from build123d import *

# Parameters (mm, degrees)
EXTRUDE_THIN1_DEPTH      = 5
EXTRUDE_THIN1_DEPTH_BACK = 1


with BuildPart() as part:
    # Sketch1 → Extrude-Thin1 (new, two sides: drawn at the far end of the back side and taken through both)
    with BuildSketch(Plane(origin=(0, 494, 0), x_dir=(1, 0, 0), z_dir=(0, 1, 0)).offset(-EXTRUDE_THIN1_DEPTH_BACK)):
        with BuildLine():
            Line((-21.192485275, 22.077376905), (159.5, 22.077376905))
            ThreePointArc((159.5, 22.077376905), (164.149331935, 20.119811555), (165.998241995, 15.426211538))
            Line((165.998241995, 15.426211538), (160.501622773, -220.860462738))
            ThreePointArc((160.501622773, -220.860462738), (166.44500383, -226.999747946), (172.499927204, -220.970444157))
            Line((172.499927204, -220.970444157), (170.499896872, 185.041870778))
            ThreePointArc((170.499896872, 185.041870778), (167.995585809, 191.02519301), (162, 193.5))
            Line((162, 193.5), (-162, 193.5))
            ThreePointArc((-162, 193.5), (-168.057344942, 190.963100892), (-170.498955066, 184.866722883))
            Line((-170.498955066, 184.866722883), (-167.998955066, 25.444099787))
            ThreePointArc((-167.998955066, 25.444099787), (-165.463100892, 19.520031962), (-159.5, 17.077376905))
            Line((-159.5, 17.077376905), (-45.192485275, 17.077376905))
            Line((-45.192485275, 17.077376905), (-45.192485275, 19.077376905))
            Line((-45.192485275, 19.077376905), (-159.5, 19.077376905))
            ThreePointArc((-159.5, 19.077376905), (-164.060018329, 20.945289596), (-165.999200933, 25.475459109))
            Line((-165.999200933, 25.475459109), (-168.499200933, 184.898082204))
            ThreePointArc((-168.499200933, 184.898082204), (-166.632087309, 189.560018329), (-162, 191.5))
            Line((-162, 191.5), (162, 191.5))
            ThreePointArc((162, 191.5), (166.584859736, 189.607500537), (168.499921138, 185.03201883))
            Line((168.499921138, 185.03201883), (170.499951469, -220.980296104))
            ThreePointArc((170.499951469, -220.980296104), (166.463335887, -224.999831964), (162.501081849, -220.906975159))
            Line((162.501081849, -220.906975159), (167.997701071, 15.379699117))
            ThreePointArc((167.997701071, 15.379699117), (165.579895607, 21.517483756), (159.5, 24.077376905))
            Line((159.5, 24.077376905), (-21.192485275, 24.077376905))
            Line((-21.192485275, 24.077376905), (-21.192485275, 22.077376905))
        make_face()
    extrude(amount=EXTRUDE_THIN1_DEPTH + EXTRUDE_THIN1_DEPTH_BACK)


solid = part.part
The listing builds one solid part. Answer for the finished solid, in the listing's coordinates (mm). Coordinates: 2 decimals unless noted, no trailing zeros. Loops run counter-clockwise (first coordinate to the right, second up) from the corner with the lowest first, then second, coordinate; pieces in that order, holes last. Notation, with made-up numbers: (-8, 79.25) -> (50, 79.25) arc R9 cw to (50, 85.25) -> close; hole circle Ø8 at (50.25, 58). An arc over 180 degrees is marked (long way). Write item = value, one per line. Start each with the question number.
1) The mould has two halves that part along X. Classify faces 1 (the face through (165.646, 495.958, -21.449)), 2 (the face through (-167.99, 495.96, -191.03)), 3 (the face through (168.06, 495.96, -190.96)): released by +X, released by -X, zero draft, split by the parting line, or undercut.
2) A cutting plane is placed at A-A (x = 129). Give the vertices of the cut face in (y, z).
3) Straight lines are drawn through the part: line 1 (Z direction, x = 99, y = 498.25); line 2 (Z direction, x = -85, y = 494.65); line 3 (X direction, y = 495.3, z = -29). For each, find the intervals that lie inside material, in ascending order. Write a range as from..to.
4) A cutting plane is placed at C-C (z = -123). Give the vertices of the cut face in (x, y).
5) Given pin 1 Ø1.8 at (x, y) = (-116.5, 496) entering from +Z; pin 2 Ø1.8 at (x, y) = (66.5, 496) entering from +Z; pin 3 Ø1 at (y, z) = (497, -18.5) entering from +X, each flat-ended and moving along its own axis, determine where each tip first touches the part or whether it passes through.
6) A cutting plane is placed at D-D (x = -35). Give the vertices of the cut face in (y, z), then the cut area to 3 significant figures.
7) A cutting plane is placed at B-B (y = 495.25). Give the vertices of the cut face in (x, z), then the cut area to 3 significant figures.
Responses:
q1.face_1 = undercut
q1.face_2 = released by -X
q1.face_3 = released by +X
q2.outline = (493, -193.5) -> (499, -193.5) -> (499, -191.5) -> (493, -191.5) -> close; (493, -24.08) -> (499, -24.08) -> (499, -22.08) -> (493, -22.08) -> close
q3.line_1 = -193.5..-191.5, -24.08..-22.08
q3.line_2 = -193.5..-191.5, -19.08..-17.08
q3.line_3 = -168.05..-166.05, 169.27..171.27
q4.outline = (-169.53, 493) -> (-167.53, 493) -> (-167.53, 499) -> (-169.53, 499) -> close; (168.81, 493) -> (170.81, 493) -> (170.81, 499) -> (168.81, 499) -> close
q5.pin_1 = -17.08
q5.pin_2 = -22.08
q5.pin_3 = 171.32
q6.outline = (493, -193.5) -> (499, -193.5) -> (499, -191.5) -> (493, -191.5) -> close
q6.area = 12.0 mm²
q7.outline = (-170.5, -184.87) arc R8.5 ccw to (-162, -193.5) -> (162, -193.5) arc R8.5 ccw to (170.5, -185.04) -> (172.5, 220.97) arc R6 ccw (long way) to (160.5, 220.86) -> (166, -15.43) arc R6.5 cw to (159.5, -22.08) -> (-21.19, -22.08) -> (-21.19, -24.08) -> (159.5, -24.08) arc R8.5 ccw to (168, -15.38) -> (162.5, 220.91) arc R4 cw (long way) to (170.5, 220.98) -> (168.5, -185.03) arc R6.5 cw to (162, -191.5) -> (-162, -191.5) arc R6.5 cw to (-168.5, -184.9) -> (-166, -25.48) arc R6.5 cw to (-159.5, -19.08) -> (-45.19, -19.08) -> (-45.19, -17.08) -> (-159.5, -17.08) arc R8.5 ccw to (-168, -25.44) -> close
q7.area = 2,970 mm²
